Geometry: see drawing. Coordinates: mm, zero at the bounding-box minimum. A direction names the side the tool comes from. Coordinates: 2 decimals unless noted, no trailing zeros. Write each loop counter-clockwise with the first axis right and the second up, starting at its lowest first coordinate (ties: lowest second). Pieces come first, ordered by that corner, then holes. Notation, with made-up numbers: (-20.75, 29) - (31.25, 29) arc R23 cw to (31.25, 43) - close; hole circle Ø6 at (77, 48.25). An arc over 180 degrees is marked (long way). Use a Markdown table: item, result. Add a question column.
Q1. Section query D-D (y = 60). Return the cut outline in (x, z).
Q2. Section query A-A (y = 37). Return the cut outline in (x, z).
Q3. Section query B-B (x = 20). Return the cut outline in (y, z).
Q4. Section query C-C (z = 7.5). Return the cut outline in (x, y), then the cut area to 3 significant figures.
Q5. Mould query, pull axis X, two halves, no side actions, for the marked faces 1, 2 and 3. Classes: released by +X, released by -X, zero draft, split by the parting line, or undercut.
Q6. Material intervals for probe 1 along X at (y, z) = (30, 7.5); probe 2 along X at (y, z) = (14.5, 7.5); probe 3 along X at (y, z) = (26, 12.5), sorted ascending. Write a range as from..to.
Q7. Pin query (flat end, axial travel): P1, Ø2, axis at x = 15, z = 7, coming from the -Y side; P2, Ø14.5, axis at x = 20, y = 60, coming from the +Z side. Return the tip coordinate at first contact, or that it passes through.
Q8. Set-up query: the marked faces 4, 5 and 6. Return all of +Z, -Z, +X, -X, +Y, -Y with unobstructed straight access to the full face (end or side cutting, diameter ignored); none if empty.
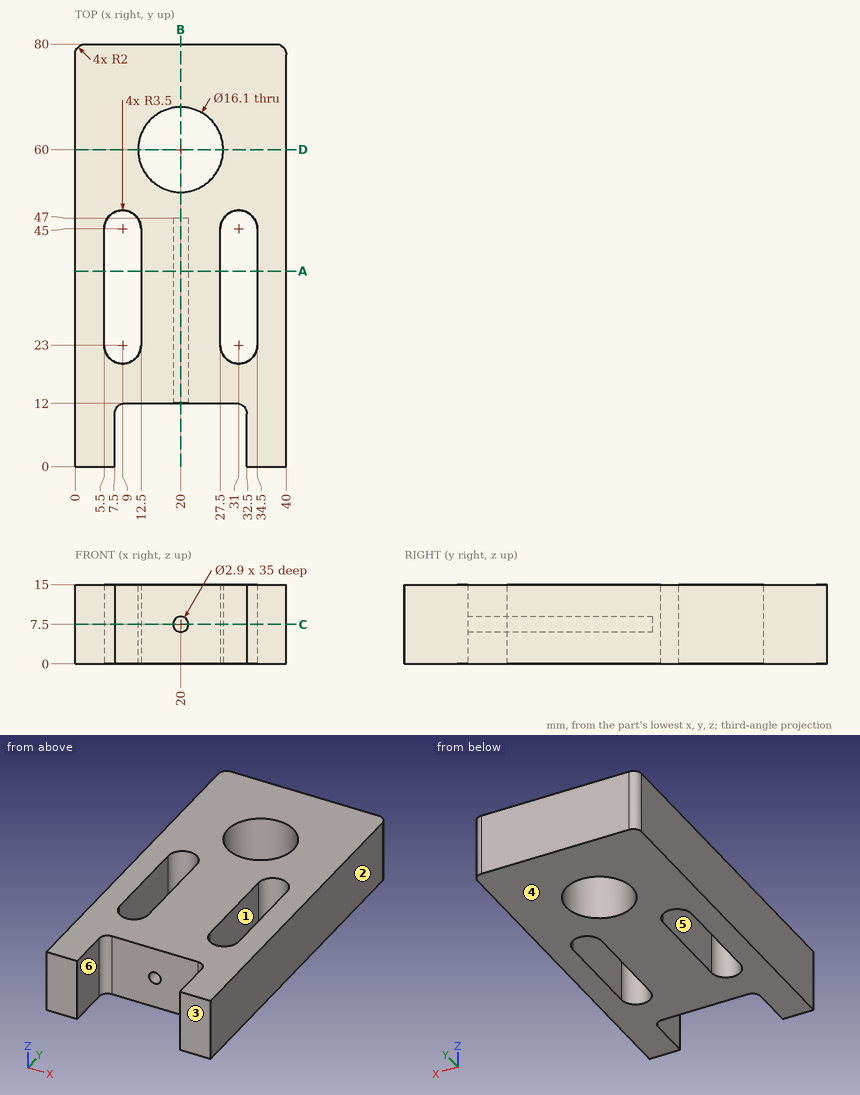
Values follow:
| question | item | result |
|---|---|---|
| 1 | outline | (0, 0) - (11.95, 0) - (11.95, 15) - (0, 15) - close; (28.05, 0) - (40, 0) - (40, 15) - (28.05, 15) - close |
| 2 | outline | (0, 0) - (5.5, 0) - (5.5, 15) - (0, 15) - close; (12.5, 0) - (27.5, 0) - (27.5, 15) - (12.5, 15) - close; (34.5, 0) - (40, 0) - (40, 15) - (34.5, 15) - close; hole circle Ø2.9 at (20, 7.5) |
| 3 | outline | (12, 0) - (51.95, 0) - (51.95, 15) - (12, 15) - (12, 8.95) - (47, 8.95) - (47, 6.05) - (12, 6.05) - close; (68.05, 0) - (80, 0) - (80, 15) - (68.05, 15) - close |
| 4 | outline | (0, 0) - (7.5, 0) - (7.5, 10) arc R2 cw to (9.5, 12) - (18.55, 12) - (18.55, 47) - (21.45, 47) - (21.45, 12) - (30.5, 12) arc R2 cw to (32.5, 10) - (32.5, 0) - (40, 0) - (40, 78) arc R2 ccw to (38, 80) - (2, 80) arc R2 ccw to (0, 78) - close; hole (5.5, 23) arc R3.5 ccw to (12.5, 23) - (12.5, 45) arc R3.5 ccw to (5.5, 45) - close; hole circle Ø16.1 at (20, 60); hole (27.5, 23) arc R3.5 ccw to (34.5, 23) - (34.5, 45) arc R3.5 ccw to (27.5, 45) - close |
| 4 | area | 2,210 mm2 |
| 5 | face 1 | undercut |
| 5 | face 2 | released by +X |
| 5 | face 3 | zero draft |
| 6 | probe 1 | 0..5.5, 12.5..18.55, 21.45..27.5, 34.5..40 |
| 6 | probe 2 | 0..18.55, 21.45..40 |
| 6 | probe 3 | 0..5.5, 12.5..27.5, 34.5..40 |
| 7 | P1 | y = 12 |
| 7 | P2 | through |
| 8 | face 4 | -Z, +X, -X, +Y, -Y |
| 8 | face 5 | +Z, -Z |
| 8 | face 6 | +Z, -Z, -Y |
